Source: CAD feature listing. Evaluate the final solid. Frame: model axes, mm. A direction names the side the tool comes from. Give positions to 0.01 mm unless a question says otherwise; leave off trailing zeros. Loops run counter-clockwise (first coordinate to the right, second up) from the corner with the lowest first, then second, coordinate; pieces in that order, holes last. Notation, with made-up numbers: (82, 13) - (115, 13) arc R26 ccw to (115, 48) - close; hole circle Ø6 at (45.25, -27). An arc over 180 degrees is marked (long way). Write each question's results on one line, items separated by ' | '. Start each with the question number.
(1) Pull-direction query (Y, two-part tool) for faces 4 (the flat face through (0, 25, 0)), 5 (the flat face through (-18, 0, -4)), 6 (the flat face through (-25, 0, 0)), 7 (the flat face through (18, 0, -4)); classes: pulls with the +Y half, pulls with the -Y half, needs draft (parallel to the pull), parting line crosses it, or undercut.
(2) Reachability of faces 1 (the flat face through (0, 0, 1.5)), 2 (the flat face through (0, -25, 0)), 3 (the flat face through (0, -18, -4)) from +Z, -Z, +X, -X, +Y, -Y: full face, straight path, thin tool, end or side. Return the list, or none.
(3) Cut plane A-A on y = -14. Return the cut outline in (x, z).
(4) Cut plane C-C on x = 6. Return the cut outline in (y, z), then the cut area to 3 significant figures.
(5) Material intervals for line 1 along X through (y, z) = (12, 5.5); line 2 along Z through (x, y) = (-3, 7.5), sorted ascending. Write a range as [from, to].
(6) Contact query for flat-ended pins moving along their axis: pin 1 (6 mm diameter, centred on x = 2.5, y = -1.5, fed in from -Z); pin 2 (12 mm diameter, centred on x = 3, y = 11.5, fed in from +Z). Output: stop coordinate, or through.
(7) Cut plane B-B on z = -5.25. Return the cut outline in (x, y), then the cut area to 3 significant figures.
from build123d import *

# Parameters (mm, degrees)
ESQUISSE1_W             = 50
ESQUISSE1_H             = 50
BOSS_EXTRU_1_DEPTH      = 6.5
BOSS_EXTRU_1_DEPTH_BACK = 6.5
ESQUISSE2_W             = 36
ESQUISSE2_H             = 36
ENL_V_MAT_EXTRU_1_DEPTH = 5
ESQUISSE3_W             = 36
ESQUISSE3_H             = 36
ENL_V_MAT_EXTRU_2_DEPTH = 5
D_GAGEMENT_M3_51_D      = 3.9


with BuildPart() as part:
    # Esquisse1 → Boss.-Extru.1 (new body, two sides)
    with BuildSketch(Plane.XY) as boss_extru_1_sk:
        Rectangle(ESQUISSE1_W, ESQUISSE1_H)
    extrude(amount=BOSS_EXTRU_1_DEPTH)
    extrude(boss_extru_1_sk.sketch, amount=-BOSS_EXTRU_1_DEPTH_BACK)

    # Esquisse2 → Enl_v. mat.-Extru.1 (cut)
    with BuildSketch(Plane.XY.offset(6.5)):
        Rectangle(ESQUISSE2_W, ESQUISSE2_H)
    extrude(amount=-ENL_V_MAT_EXTRU_1_DEPTH, mode=Mode.SUBTRACT)

    # Esquisse3 → Enl_v. mat.-Extru.2 (cut)
    with BuildSketch(Plane(origin=(0, 0, -6.5), x_dir=(-1, 0, 0), z_dir=(0, 0, -1))):
        Rectangle(ESQUISSE3_W, ESQUISSE3_H)
    extrude(amount=-ENL_V_MAT_EXTRU_2_DEPTH, mode=Mode.SUBTRACT)

    # D_gagement M3.51 (through all)
    with Locations(Plane.XY.offset(1.5)):
        with Locations((-11.313708499, 14), (11.313708499, -14)):
            Hole(D_GAGEMENT_M3_51_D / 2)


solid = part.part
Ans:
1) face 4: pulls with the +Y half | face 5: undercut | face 6: needs draft | face 7: undercut
2) face 1: +Z | face 2: +Z, -Z, +X, -X, -Y | face 3: -Z
3) outline: (-25, -6.5) - (-18, -6.5) - (-18, -1.5) - (9.36, -1.5) - (9.36, 1.5) - (-18, 1.5) - (-18, 6.5) - (-25, 6.5) - close; (13.26, -1.5) - (18, -1.5) - (18, -6.5) - (25, -6.5) - (25, 6.5) - (18, 6.5) - (18, 1.5) - (13.26, 1.5) - close
4) outline: (-25, -6.5) - (-18, -6.5) - (-18, -1.5) - (18, -1.5) - (18, -6.5) - (25, -6.5) - (25, 6.5) - (18, 6.5) - (18, 1.5) - (-18, 1.5) - (-18, 6.5) - (-25, 6.5) - close | area: 290 mm^2
5) line 1: [-25, -18], [18, 25] | line 2: [-1.5, 1.5]
6) pin 1: z = -1.5 | pin 2: z = 1.5
7) outline: (-25, -25) - (25, -25) - (25, 25) - (-25, 25) - close; hole (-18, -18) - (18, -18) - (18, 18) - (-18, 18) - close | area: 1,200 mm^2
